Autodesk Inventor part; units mm, degrees
ref_plane "YZ Plane" through (0, 0, 0) normal (1, 0, 0) x (0, 1, 0)
ref_plane "XZ Plane" through (0, 0, 0) normal (0, 1, 0) x (-1, 0, 0)
ref_plane "XY Plane" through (0, 0, 0) normal (0, 0, 1) x (1, 0, 0)
sketch "Sketch1" plane through (0, 0, 0) normal (0, 0, 1) x (1, 0, 0)
  line L0 (-3.6735, 6.3627) -> (3.6735, 6.3627)
  line L1 (3.6735, 6.3627) -> (7.347, 0)
  line L2 (7.347, 0) -> (3.6735, -6.3627)
  line L3 (3.6735, -6.3627) -> (-3.6735, -6.3627)
  line L4 (-3.6735, -6.3627) -> (-7.347, 0)
  line L5 (-7.347, 0) -> (-3.6735, 6.3627)
  line L6 (-15.4185, 0) -> (15.4185, 0) construction
  line L7 (-5.5066, 9.5377) -> (5.5066, 9.5377)
  line L8 (5.5066, 9.5377) -> (11.0132, 0)
  line L9 (11.0132, 0) -> (5.5066, -9.5377)
  line L10 (5.5066, -9.5377) -> (-5.5066, -9.5377)
  line L11 (-5.5066, -9.5377) -> (-11.0132, 0)
  line L12 (-11.0132, 0) -> (-5.5066, 9.5377)
  point P0 (0, 0)
  point P1 (0, 0)
  point P2 (0, 0)
  dimension "d0" = 12.7254
  dimension "d1" = 3.175
extrude "Extrusion1" add sketch "Sketch1" along normal blind 12.7
fillet "Fillet1" radius 3.175 6 edges at (5.5066, -9.5377, 6.35) (-5.5066, -9.5377, 6.35) (11.0132, 0, 6.35) (-11.0132, 0, 6.35) (-5.5066, 9.5377, 6.35) (5.5066, 9.5377, 6.35)
properties part number "1-2in_spacer"
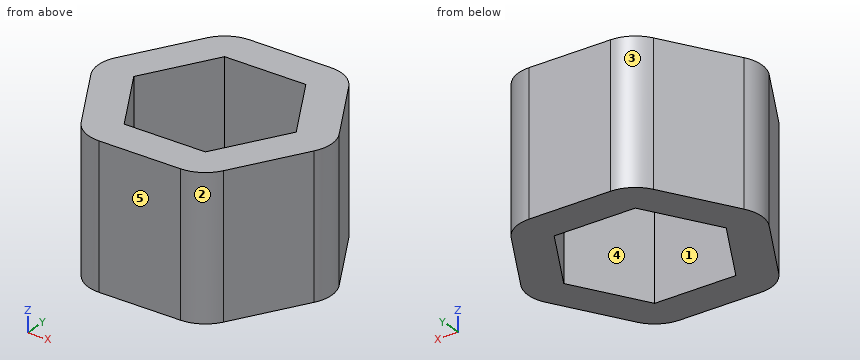
Work out the finished part from the listing and answer in its coordinate system (mm). Face numbers are marked on the shaded views. A direction names the side the tool comes from. Round coordinates to 2 decimals unless told otherwise and drop trailing zeros. Write each loop counter-clockwise with the first axis right and the second up, starting at its lowest first coordinate (ties: lowest second). Pieces come first, ordered by that corner, then holes. Notation, with made-up numbers: (-35.75, 89.5) -> (-28.75, 89.5) arc R20 cw to (-28.75, 113.5) -> close; hole circle Ø3 at (-26.5, 67.25). An arc over 180 degrees is marked (long way). Write each question's results on one line, items separated by ' | '.
Item 1: Which of the six approach directions +Z, -Z, +X, -X, +Y, -Y give full straight-line access (tool end or side, diameter ignored) to the marked faces 1 and 2?
Result set:
face 1: +Z, -Z | face 2: +Z, -Z, +X, -Y
Item 2: A cutting plane is placed at A-A, the plane x = -3. Determine the outline of the cut face in (y, z).
Result set:
outline: (-9.54, 0) -> (-6.36, 0) -> (-6.36, 12.7) -> (-9.54, 12.7) -> close; (6.36, 0) -> (9.54, 0) -> (9.54, 12.7) -> (6.36, 12.7) -> close
Item 3: A cutting plane is placed at D-D, the plane y = 8.25. Determine the outline of the cut face in (x, z).
Result set:
outline: (-6.23, 0) -> (6.23, 0) -> (6.23, 12.7) -> (-6.23, 12.7) -> close
Item 4: A cutting plane is placed at C-C, the plane y = -0.75. Determine the outline of the cut face in (x, z).
Result set:
outline: (-10.43, 0) -> (-6.91, 0) -> (-6.91, 12.7) -> (-10.43, 12.7) -> close; (6.91, 0) -> (10.43, 0) -> (10.43, 12.7) -> (6.91, 12.7) -> close
Item 5: Find the intervals of material crossed by line 1 along Y through (x, z) = (3.5, 6); line 2 along Y through (x, z) = (-6, 7.5); line 3 along X through (y, z) = (1.5, 9.25), in increasing order. Write a range as [from, to].
Result set:
line 1: [-9.54, -6.36], [6.36, 9.54] | line 2: [-8.52, -2.33], [2.33, 8.52] | line 3: [-10.15, -6.48], [6.48, 10.15]
Item 6: The mould has two halves that part along X. Classify the marked faces 3, 4 and 5: +X half, -X half, draft (parallel to the pull), parting line (faces both ways), or undercut.
Result set:
face 3: -X half | face 4: undercut | face 5: draft
Item 7: Flat-ended cylindrical pins translate along their axes: P1, Ø1, axis at x = 7.5, z = 4.5, coming from the +Y side; P2, Ø6, axis at y = 5, z = 10.5, coming from the +X side. Find the tip coordinate at first contact, or state that the pin passes through.
Result set:
P1: y = 6.95 | P2: x = 9.86
